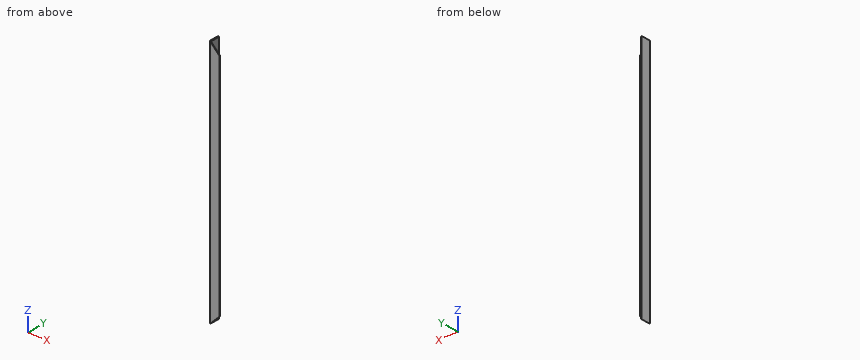
from build123d import *

# Parameters (mm, degrees)
EXTRUDE_THIN1_DEPTH = 392
CUT_EXTRUDE1_DEPTH  = 393.613041047


with BuildPart() as part:
    # Sketch1 → Extrude-Thin1 (new body)
    with BuildSketch(Plane.XY):
        Polygon((15, 0), (0, 0), (0, 15), (-1, 15), (-1, -1), (15, -1), align=None)
    extrude(amount=EXTRUDE_THIN1_DEPTH)

    # Sketch2 → Cut-Extrude1 (cut, through all)
    with BuildSketch(Plane.XZ.offset(1)):
        Polygon((-1, 392), (15, 376), (15, 392), align=None)
        Polygon((15, 16), (15, 0), (-1, 0), align=None)
    extrude(amount=-CUT_EXTRUDE1_DEPTH, mode=Mode.SUBTRACT)


solid = part.part
Can you work these out from the model? Positions are in its coordinate system, mm. Coordinates: 2 decimals unless noted, no trailing zeros. Loops run counter-clockwise (first coordinate to the right, second up) from the corner with the lowest first, then second, coordinate; pieces in that order, holes last. Notation, with made-up numbers: (79.5, 15.5) - (106.5, 15.5) arc R27 ccw to (106.5, 35.5) - close; hole circle Ø4 at (-39, -14.75). An arc over 180 degrees is marked (long way). Answer as a JSON object with one key per item and string values. Group by question number.
Item 1: For pin 1 (3 mm diameter, centred on x = 10.5, y = 2.5, fed in from -Z); pin 2 (7.5 mm diameter, centred on y = 5.5, z = 235.5, fed in from +X), each with a flat end and sliding along its axis, tell me the tip position at first contact or that it passes through.
Item 2: If we section it at A-A (x = 9.75): List the corners of the cut face in (y, z) for me.
Item 3: If I drill on L1, parallel to Y at x = 8, z = 366.5; L2, parallel to Z at x = 1.75, y = -0.25, over which ranges is the centre line in solid material (lowest first)? Write a range as from..to.
Item 4: If we section it at B-B (z = 194): List the corners of the cut face in (x, y) for me, plus the area to 3 significant figures.
Returned:
{
 "1": {"pin 1": "passes through", "pin 2": "stops at x = 0"},
 "2": {"outline": "(-1, 10.75) - (0, 10.75) - (0, 381.25) - (-1, 381.25) - close"},
 "3": {"L1": "y = -1..0", "L2": "z = 2.75..389.25"},
 "4": {"outline": "(-1, -1) - (15, -1) - (15, 0) - (0, 0) - (0, 15) - (-1, 15) - close", "area": "31.0 mm²"}
}
